Can you work these out from the model? Positions are in its coordinate system, mm. A direction names the side the tool comes from. Give positions to 0.01 mm unless a question says otherwise; leave off trailing zeros. Loops run counter-clockwise (first coordinate to the right, second up) from the corner with the lowest first, then second, coordinate; pieces in that order, holes last. Notation, with made-up numbers: (35, 3) -> (69, 3) arc R24 ccw to (69, 23) -> close; hole circle Ø5 at (49.25, -15). An arc over 180 degrees is marked (long way). One line per question, with ' | ' between items.
from build123d import *

# Parameters (mm, degrees)
SKETCH_1_W          = 18
SKETCH_1_H          = 16
EXTRUDE_1_DEPTH     = 4
SKETCH_2_R          = 1.65
CUT_EXTRUDE_1_DEPTH = 4
EXTRUDE_2_DEPTH     = 4
SKETCH_4_W          = 18
SKETCH_4_H          = 4
EXTRUDE_3_DEPTH     = 100
EXTRUDE_4_DEPTH     = 2
SKETCH_6_R          = 1.65
CUT_EXTRUDE_2_DEPTH = 10
SKETCH_7_W          = 18
SKETCH_7_H          = 7
CUT_EXTRUDE_3_DEPTH = 10
CHAMFER_1_SIZE      = 4


with BuildPart() as part:
    # 草图1 → 凸台-拉伸1 (new body)
    with BuildSketch(Plane(origin=(0, 0, 0), x_dir=(1, 0, 0), z_dir=(0, 1, 0))):
        Rectangle(SKETCH_1_W, SKETCH_1_H)
    extrude(amount=EXTRUDE_1_DEPTH)

    # 草图2 → 切除-拉伸1 (cut)
    with BuildSketch(Plane(origin=(0, 4, 0), x_dir=(1, 0, 0), z_dir=(0, 1, 0))):
        with Locations(Location((0, 0, 0), (0, 0, 270))):
            Circle(SKETCH_2_R)
    extrude(amount=-CUT_EXTRUDE_1_DEPTH, mode=Mode.SUBTRACT)

    # 草图3 → 凸台-拉伸2 (add)
    with BuildSketch(Plane(origin=(0, 4, 0), x_dir=(1, 0, 0), z_dir=(0, 1, 0))):
        Polygon((-9, -8), (-9, -12), (-7, -12), (-4, -8), align=None)
        Polygon((7, -12), (4, -8), (9, -8), (9, -12), align=None)
        Polygon((9, 12), (7, 12), (4, 8), (9, 8), align=None)
        Polygon((-7, 12), (-4, 8), (-9, 8), (-9, 12), align=None)
    extrude(amount=-EXTRUDE_2_DEPTH)

    # 草图4 → 凸台-拉伸3 (add)
    with BuildSketch(Plane(origin=(0, 4, 0), x_dir=(1, 0, 0), z_dir=(0, 1, 0))):
        with Locations((0, -6)):
            Rectangle(SKETCH_4_W, SKETCH_4_H)
    extrude(amount=EXTRUDE_3_DEPTH)

    # 草图5 → 凸台-拉伸4 (add)
    with BuildSketch(Plane(origin=(9, 0, 0), x_dir=(0, 0, -1), z_dir=(1, 0, 0))):
        Polygon((-4, 19), (-4, 4), (4, 4), align=None)
        Polygon((-8, 12), (-8, 4), (-12, 4), align=None)
    extrude_4 = extrude(amount=-EXTRUDE_4_DEPTH)

    # 镜向1: 凸台-拉伸4 across plane
    add(extrude_4.mirror(Plane(origin=(0, 0, 0), x_dir=(0, 0, 1), z_dir=(1, 0, 0))))

    # 草图6 → 切除-拉伸2 (cut)
    with BuildSketch(Plane(origin=(0, 0, 4), x_dir=(-1, 0, 0), z_dir=(0, 0, -1))):
        with Locations((-6, 44)):
            Circle(SKETCH_6_R)
        with Locations((6, 44)):
            Circle(SKETCH_6_R)
        with Locations((6, 64)):
            Circle(SKETCH_6_R)
        with Locations((-6, 64)):
            Circle(SKETCH_6_R)
        with Locations((6, 24)):
            Circle(SKETCH_6_R)
        with Locations((-6, 24)):
            Circle(SKETCH_6_R)
        with Locations((5, 92)):
            Circle(SKETCH_6_R)
        with Locations((5, 86)):
            Circle(SKETCH_6_R)
        with Locations((5, 80)):
            Circle(SKETCH_6_R)
        with Locations((5, 74)):
            Circle(SKETCH_6_R)
        with Locations((5, 68)):
            Circle(SKETCH_6_R)
        with Locations((5, 56)):
            Circle(SKETCH_6_R)
        with Locations((5, 50)):
            Circle(SKETCH_6_R)
        with Locations((-5, 50)):
            Circle(SKETCH_6_R)
        with Locations((-5, 56)):
            Circle(SKETCH_6_R)
        with Locations((-5, 68)):
            Circle(SKETCH_6_R)
        with Locations((-5, 74)):
            Circle(SKETCH_6_R)
        with Locations((-5, 80)):
            Circle(SKETCH_6_R)
        with Locations((-5, 86)):
            Circle(SKETCH_6_R)
        with Locations((-5, 92)):
            Circle(SKETCH_6_R)
    extrude(amount=-CUT_EXTRUDE_2_DEPTH, mode=Mode.SUBTRACT)

    # 草图7 → 切除-拉伸3 (cut)
    with BuildSketch(Plane(origin=(0, 0, 4), x_dir=(-1, 0, 0), z_dir=(0, 0, -1))):
        with Locations((0, 100.5)):
            Rectangle(SKETCH_7_W, SKETCH_7_H)
    extrude(amount=-CUT_EXTRUDE_3_DEPTH, mode=Mode.SUBTRACT)

    # 倒角1
    chamfer_1_edges = [part.edges().sort_by_distance(p)[0] for p in [
        (-9, 97, 6),
        (9, 97, 6),
    ]]
    chamfer(chamfer_1_edges, length=CHAMFER_1_SIZE)


solid = part.part
Q1. On a 3-axis mill with a long thin cutter (end or side, diameter ignored), from which of +Z, -Z, +X, -X, +Y, -Y can I reach the whole of each face in a straight line? I mean faces 1 (the face through (5.5, 2, 10)), 2 (the face through (7, 6, 9)), 3 (the face through (0, 50, 4)). Say none if no direction works.
Entries:
face 1: +Z, +Y, -Y | face 2: +Z, +Y | face 3: -Z, +Y
Q2. For pin 1 Ø2.5 at (x, y) = (6, 64) entering from +Z; pin 2 Ø3 at (x, y) = (1, 36) entering from +Z; pin 3 Ø3 at (x, y) = (1, 66) entering from -Z; pin 4 Ø5 at (x, z) = (-0.5, -2) entering from +Y, each with a flat end and sliding along its axis, tell me the tip position at first contact or that it passes through.
Entries:
pin 1: through | pin 2: z = 8 | pin 3: z = 4 | pin 4: y = 4
Q3. If we section it at B-B (y = 68): Write out the boundary of the cut face in (x, z).
Entries:
outline: (-9, 4) -> (-6.65, 4) -> (-6.65, 8) -> (-9, 8) -> close; (-3.35, 4) -> (3.35, 4) -> (3.35, 8) -> (-3.35, 8) -> close; (6.65, 4) -> (9, 4) -> (9, 8) -> (6.65, 8) -> close
Q4. If I drill on probe 1 along X at (y, z) = (68, 6.75); probe 2 along Z at (x, y) = (-1.5, 13); probe 3 along Y at (x, z) = (4.25, -3), over which ranges is the centre line in solid material (lowest first)? Write a range as from..to.
Entries:
probe 1: -9..-6.65, -3.35..3.35, 6.65..9 | probe 2: 4..8 | probe 3: 0..4
Q5. If we mould it in two halves opening along X, with no side actions, what happens to faces 4 (the face through (8, 2, 12)), 5 (the face through (-4.6, 78.4, 6)), 6 (the face through (9, 33, 5))? For each: pulls with the +X half, pulls with the -X half, needs draft (parallel to the pull), parting line crosses it, or undercut.
Entries:
face 4: needs draft | face 5: undercut | face 6: pulls with the +X half
Q6. If we section it at A-A (z = 0): Write out the boundary of the cut face in (x, y), plus the area to 3 significant figures.
Entries:
outline: (-9, 0) -> (-1.65, 0) -> (-1.65, 4) -> (-7, 4) -> (-7, 11.5) -> (-9, 11.5) -> close; (1.65, 0) -> (9, 0) -> (9, 11.5) -> (7, 11.5) -> (7, 4) -> (1.65, 4) -> close | area: 88.8 mm²
Q7. If we section it at C-C (y = 38): Write out the boundary of the cut face in (x, z).
Entries:
outline: (-9, 4) -> (9, 4) -> (9, 8) -> (-9, 8) -> close
